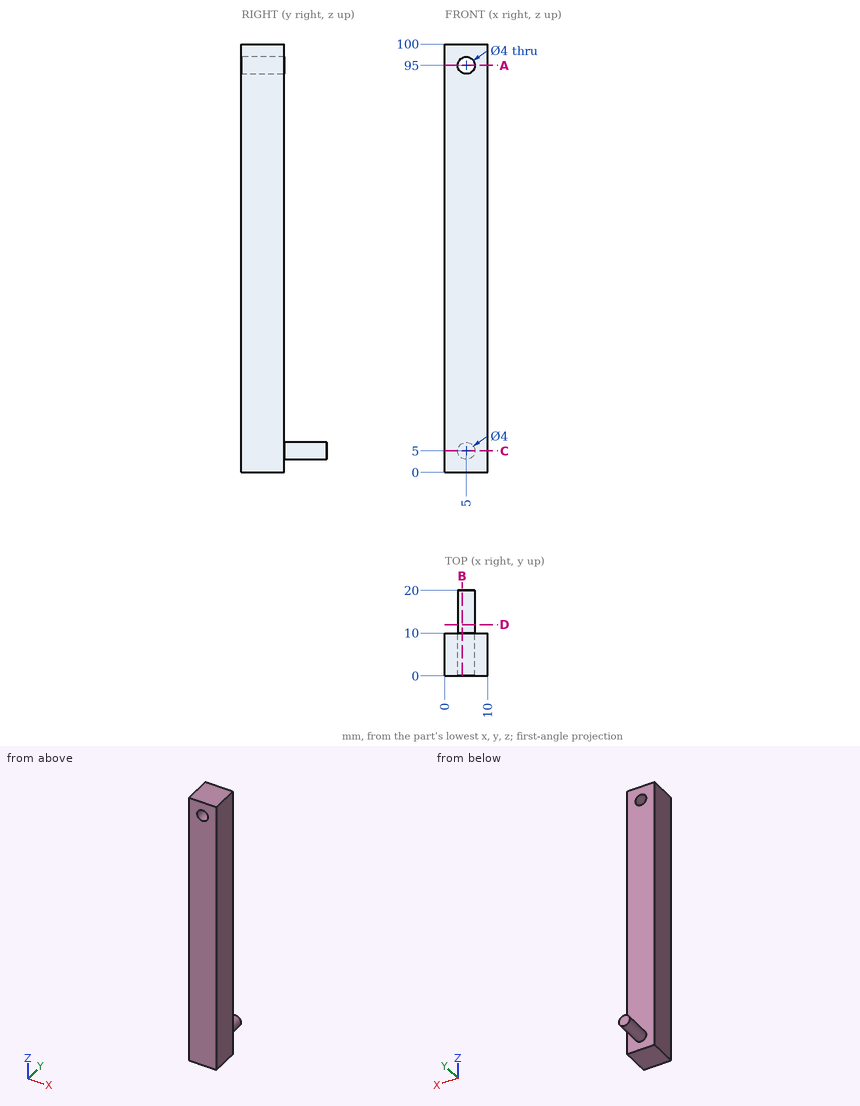
Here's the drawing with two shaded views (mm, measured from the low corner). I have some questions. Give positions to 0.01 mm unless a question says otherwise; leave off trailing zeros. Loops run counter-clockwise (first coordinate to the right, second up) from the corner with the lowest first, then second, coordinate; pieces in that order, holes last. Notation, with made-up numbers: M 31.5,5.5 L 58.5,5.5 A21 ccw 58.5,34.5 Z; hole C 88.5,-18.5 d7. An arc over 180 degrees is marked long. Use one line per item in the form item = value. Start each with the question number.
(1) I want a section at A-A, the plane z = 95. Write out the boundary of the cut face in (x, y), and give its area (3 significant figures).
(2) Please list where these lines run through material, in increasing order: line 1 (X direction, y = 6, z = 95); line 2 (Y direction, x = 0.5, z = 16.5); line 3 (Z direction, x = 5.5, y = 9.5).
(3) I'm going to push a flat-ended pin straight in: P1, Ø3, axis at x = 7.5, z = 84, coming from the +Y side. Where does the tip first touch, or does it pass through?
(4) I want a section at D-D, the plane y = 12. Write out the boundary of the cut face in (x, z).
(5) I want a section at B-B, the plane x = 4. Write out the boundary of the cut face in (y, z).
(6) I want a section at C-C, the plane z = 5. Write out the boundary of the cut face in (x, y), and give its area (3 significant figures).
Worked out:
q1.outline = M 0,0 L 3,0 L 3,10 L 0,10 Z; M 7,0 L 10,0 L 10,10 L 7,10 Z
q1.area = 60.0 mm²
q2.line_1 = 0 to 3, 7 to 10
q2.line_2 = 0 to 10
q2.line_3 = 0 to 93.06, 96.94 to 100
q3.P1 = 10
q4.outline = C 5,5 d4
q5.outline = M 0,0 L 10,0 L 10,3.27 L 20,3.27 L 20,6.73 L 10,6.73 L 10,93.27 L 0,93.27 Z; M 0,96.73 L 10,96.73 L 10,100 L 0,100 Z
q6.outline = M 0,0 L 10,0 L 10,10 L 7,10 L 7,20 L 3,20 L 3,10 L 0,10 Z
q6.area = 140 mm²
